Geometry check sheet. Reference: the model listing, model coordinates, mm. Face numbers are marked on the shaded views. Coordinates: 2 decimals unless noted, no trailing zeros. Order: outer loops, then holes, each group sorted by start corner. A loop starts at its lowest first (then second) coordinate and runs counter-clockwise, first axis right, second up.
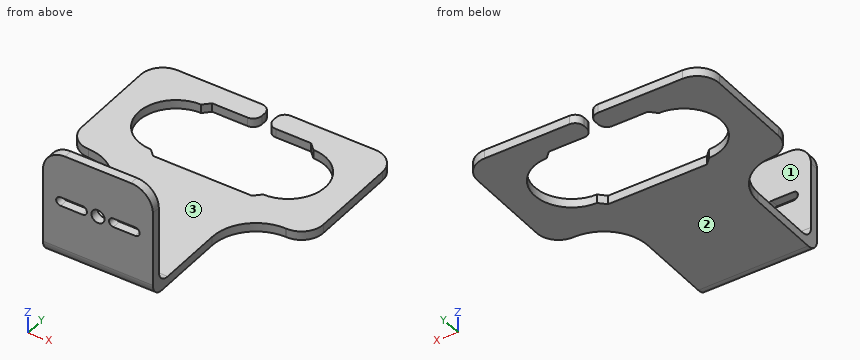
```python
from build123d import *

# Parameters (mm, degrees)
BOSS_EXTRUDE1_DEPTH = 2
SKETCH2_W           = 25
SKETCH2_H           = 2
BOSS_EXTRUDE2_DEPTH = 23
FILLET1_R           = 3
FILLET2_R           = 10
FILLET3_R           = 5
SKETCH3_R           = 1.5
CUT_EXTRUDE1_DEPTH  = 2


with BuildPart() as part:
    # Sketch1 → Boss-Extrude1 (new body)
    with BuildSketch(Plane.XY):
        with BuildLine():
            Line((-1.333510856, 27.908436521), (-1.333510856, 26.904337049))
            ThreePointArc((-1.333510856, 26.904337049), (-1.919297294, 25.490123487), (-3.333510856, 24.904337049))
            Line((-3.333510856, 24.904337049), (-11.337610328, 24.904337049))
            Line((-11.337610328, 24.904337049), (-12.833510856, 23.408436521))
            ThreePointArc((-12.833510856, 23.408436521), (-21.333510856, 14.908436521), (-12.833510856, 6.408436521))
            Line((-12.833510856, 6.408436521), (-11.329411385, 4.904337049))
            Line((-11.329411385, 4.904337049), (11.162389672, 4.904337049))
            Line((11.162389672, 4.904337049), (12.666489144, 6.408436521))
            ThreePointArc((12.666489144, 6.408436521), (21.166489144, 14.908436521), (12.666489144, 23.408436521))
            Line((12.666489144, 23.408436521), (11.170588615, 24.904337049))
            Line((11.170588615, 24.904337049), (3.166489144, 24.904337049))
            ThreePointArc((3.166489144, 24.904337049), (1.752275581, 25.490123487), (1.166489144, 26.904337049))
            Line((1.166489144, 26.904337049), (1.166489144, 27.908436521))
            ThreePointArc((1.166489144, 27.908436521), (1.752275581, 29.322650083), (3.166489144, 29.908436521))
            Line((3.166489144, 29.908436521), (22.416489144, 29.908436521))
            ThreePointArc((22.416489144, 29.908436521), (25.95202305, 28.443970427), (27.416489144, 24.908436521))
            Line((27.416489144, 24.908436521), (27.416489144, 4.904337049))
            ThreePointArc((27.416489144, 4.904337049), (25.95202305, 1.368803144), (22.416489144, -0.095662951))
            Line((22.416489144, -0.095662951), (12.166489144, -0.095662951))
            Line((12.166489144, -0.095662951), (12.166489144, -30.091563479))
            Line((12.166489144, -30.091563479), (-12.833510856, -30.091563479))
            Line((-12.833510856, -30.091563479), (-12.833510856, -0.095662951))
            Line((-12.833510856, -0.095662951), (-22.583510856, -0.095662951))
            ThreePointArc((-22.583510856, -0.095662951), (-26.119044762, 1.368803144), (-27.583510856, 4.904337049))
            Line((-27.583510856, 4.904337049), (-27.583510856, 24.908436521))
            ThreePointArc((-27.583510856, 24.908436521), (-26.119044762, 28.443970427), (-22.583510856, 29.908436521))
            Line((-22.583510856, 29.908436521), (-3.333510856, 29.908436521))
            ThreePointArc((-3.333510856, 29.908436521), (-1.919297294, 29.322650083), (-1.333510856, 27.908436521))
        make_face()
    extrude(amount=-BOSS_EXTRUDE1_DEPTH)

    # Sketch2 → Boss-Extrude2 (add)
    with BuildSketch(Plane.XY):
        with Locations((-0.333510856, -29.091563479)):
            Rectangle(SKETCH2_W, SKETCH2_H)
    extrude(amount=BOSS_EXTRUDE2_DEPTH)

    # Fillet1
    fillet1_edges = [part.edges().sort_by_distance(p)[0] for p in [
        (-0.333510856, -30.091563479, -2),
        (-0.333510856, -28.091563479, 0),
    ]]
    fillet(fillet1_edges, radius=FILLET1_R)

    # Fillet2
    fillet2_edges = [part.edges().sort_by_distance(p)[0] for p in [
        (-12.833510856, -0.095662951, -1),
        (12.166489144, -0.095662951, -1),
    ]]
    fillet(fillet2_edges, radius=FILLET2_R)

    # Fillet3
    fillet3_edges = [part.edges().sort_by_distance(p)[0] for p in [
        (-12.833510856, -29.091563479, 23),
        (12.166489144, -29.091563479, 23),
    ]]
    fillet(fillet3_edges, radius=FILLET3_R)

    # Sketch3 → Cut-Extrude1 (cut)
    with BuildSketch(Plane.XZ.offset(30.091563479)):
        with Locations((-0.333510856, 12)):
            Circle(SKETCH3_R)
        with BuildLine():
            Line((3.166489144, 11), (8.166489144, 11))
            ThreePointArc((8.166489144, 11), (9.166489144, 12), (8.166489144, 13))
            Line((8.166489144, 13), (3.166489144, 13))
            ThreePointArc((3.166489144, 13), (2.166489144, 12), (3.166489144, 11))
        make_face()
        with BuildLine():
            Line((-3.833510856, 13), (-8.833510856, 13))
            ThreePointArc((-8.833510856, 13), (-9.833510856, 12), (-8.833510856, 11))
            Line((-8.833510856, 11), (-3.833510856, 11))
            ThreePointArc((-3.833510856, 11), (-2.833510856, 12), (-3.833510856, 13))
        make_face()
    extrude(amount=-CUT_EXTRUDE1_DEPTH, mode=Mode.SUBTRACT)


solid = part.part
```
Item 1: Release check for a two-part mould opening along Z. For the marked faces 1, 2 and 3 record: pulls with the +Z half, pulls with the -Z half, needs draft (parallel to the pull), parting line crosses it, or undercut.
Item 2: Depth check by flat-ended pin: P1, Ø0.8, axis at y = 27.5, z = -1, coming from the +X side; P2, Ø0.6, axis at x = 8.5, z = -0.5, coming from the -Y side; P3, Ø6, axis at x = -12, y = -10, coming from the +Z side. Enter the tip coordinate at first touch or a pass-through.
Item 3: Sectioned sample at A-A (z = 12). Record the cut outline in (x, y), and give its area (3 significant figures).
Item 4: Thickness scan on line 1 along Z through (x, y) = (-2, -6.5); line 2 along Y through (x, z) = (-11.5, 9.75). Record the ranges inside material, lowest first.
Item 5: Sectioned sample at C-C (z = 8). Record the cut outline in (x, y), and give its area (3 significant figures).
Item 6: Sectioned sample at B-B (y = -11.5). Record the cut outline in (x, z).
Geometry check:
1. face 1: needs draft
1. face 2: pulls with the -Z half
1. face 3: pulls with the +Z half
2. P1: stops at x = 26.91
2. P2: stops at y = -29.84
2. P3: stops at z = 0
3. outline: (-12.83, -30.09) - (-9.83, -30.09) - (-9.83, -28.09) - (-12.83, -28.09) - close; (-2.83, -30.09) - (-1.83, -30.09) - (-1.83, -28.09) - (-2.83, -28.09) - close; (1.17, -30.09) - (2.17, -30.09) - (2.17, -28.09) - (1.17, -28.09) - close; (9.17, -30.09) - (12.17, -30.09) - (12.17, -28.09) - (9.17, -28.09) - close
3. area: 16.0 mm2
4. line 1: z = -2 to 0
4. line 2: y = -30.09 to -28.09
5. outline: (-12.83, -30.09) - (12.17, -30.09) - (12.17, -28.09) - (-12.83, -28.09) - close
5. area: 50.0 mm2
6. outline: (-12.83, -2) - (12.17, -2) - (12.17, 0) - (-12.83, 0) - close
